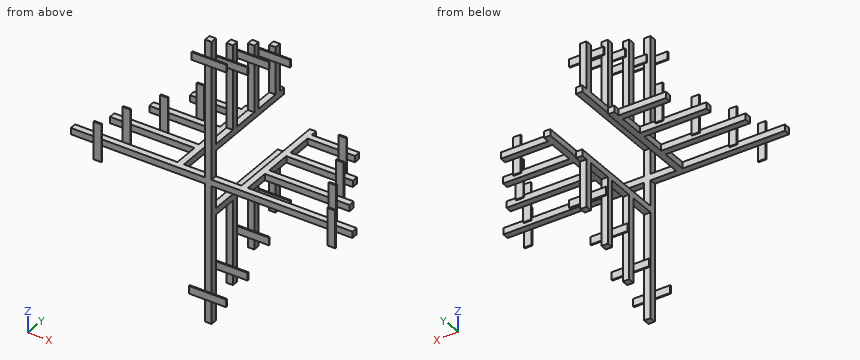
from build123d import *

# Parameters (mm, degrees)
SKETCH3_W                 = 25
SKETCH3_H                 = 25
BOSS_EXTRUDE2_DEPTH       = 550
SKETCH5_W                 = 25
SKETCH5_H                 = 25
BOSS_EXTRUDE3_DEPTH       = 550
SKETCH7_W                 = 25
SKETCH7_H                 = 25
BOSS_EXTRUDE4_DEPTH       = 400
SKETCH8_W                 = 25
SKETCH8_H                 = 25
BOSS_EXTRUDE5_DEPTH       = 400
SKETCH9_W                 = 25
SKETCH9_H                 = 25
BOSS_EXTRUDE7_DEPTH       = 260
SKETCH9_5_W               = 25
SKETCH9_5_H               = 25
BOSS_EXTRUDE8_DEPTH       = 330
SKETCH9_8_W               = 25
SKETCH9_8_H               = 25
BOSS_EXTRUDE10_DEPTH      = 185
SKETCH11_W                = 25
SKETCH11_H                = 25
BOSS_EXTRUDE11_DEPTH      = 185
SKETCH11_5_W              = 25
SKETCH11_5_H              = 25
BOSS_EXTRUDE12_DEPTH      = 260
SKETCH11_6_W              = 25
SKETCH11_6_H              = 25
BOSS_EXTRUDE13_DEPTH      = 330
SKETCH12_W                = 25
SKETCH12_H                = 25
BOSS_EXTRUDE14_DEPTH      = 185
SKETCH12_3_W              = 25
SKETCH12_3_H              = 25
BOSS_EXTRUDE15_DEPTH      = 260
SKETCH12_4_W              = 25
SKETCH12_4_H              = 25
BOSS_EXTRUDE16_DEPTH      = 330
SKETCH13_W                = 25
SKETCH13_H                = 25
BOSS_EXTRUDE17_DEPTH      = 330
SKETCH13_3_W              = 25
SKETCH13_3_H              = 25
BOSS_EXTRUDE18_DEPTH      = 260
SKETCH13_4_W              = 25
SKETCH13_4_H              = 25
BOSS_EXTRUDE19_DEPTH      = 185
BOSS_EXTRUDE21_DEPTH      = 61
BOSS_EXTRUDE21_DEPTH_BACK = 75
SKETCH15_W                = 30
SKETCH15_H                = 5
BOSS_EXTRUDE22_DEPTH      = 60
BOSS_EXTRUDE22_DEPTH_BACK = 75
SKETCH16_W                = 30
SKETCH16_H                = 5
BOSS_EXTRUDE23_DEPTH      = 61
BOSS_EXTRUDE23_DEPTH_BACK = 86
SKETCH18_W                = 30
SKETCH18_H                = 5
BOSS_EXTRUDE24_DEPTH      = 60
BOSS_EXTRUDE24_DEPTH_BACK = 85
SKETCH19_W                = 30
SKETCH19_H                = 5
BOSS_EXTRUDE27_DEPTH      = 61
BOSS_EXTRUDE27_DEPTH_BACK = 86
SKETCH20_W                = 30
SKETCH20_H                = 5


with BuildPart() as part:
    # Sketch3 → Boss-Extrude2 (new, symmetric)
    with BuildSketch(Plane.XY):
        Rectangle(SKETCH3_W, SKETCH3_H)
    extrude(amount=BOSS_EXTRUDE2_DEPTH, both=True)

    # Sketch5 → Boss-Extrude3 (add, symmetric)
    with BuildSketch(Plane(origin=(12.5, 0, 0), x_dir=(0, 0, -1), z_dir=(1, 0, 0))):
        Rectangle(SKETCH5_W, SKETCH5_H)
    extrude(amount=BOSS_EXTRUDE3_DEPTH, both=True)

    # Sketch7 → Boss-Extrude4 (add)
    with BuildSketch(Plane(origin=(0, 12.5, 0), x_dir=(1, 0, 0), z_dir=(0, 1, 0))):
        with Locations((0, -125)):
            Rectangle(SKETCH7_W, SKETCH7_H)
        with Locations((0, 125)):
            Rectangle(SKETCH7_W, SKETCH7_H)
    extrude(amount=BOSS_EXTRUDE4_DEPTH)

    # Sketch8 → Boss-Extrude5 (add)
    with BuildSketch(Plane(origin=(0, 12.5, 0), x_dir=(1, 0, 0), z_dir=(0, 1, 0))):
        with Locations((125, 0)):
            Rectangle(SKETCH8_W, SKETCH8_H)
        with Locations((-125, 0)):
            Rectangle(SKETCH8_W, SKETCH8_H)
    extrude(amount=BOSS_EXTRUDE5_DEPTH)

    # Sketch9 → Boss-Extrude7 (add)
    with BuildSketch(Plane.XY.offset(137.5)):
        with Locations((0, 250)):
            Rectangle(SKETCH9_W, SKETCH9_H)
    extrude(amount=BOSS_EXTRUDE7_DEPTH)

    # Sketch9<5> → Boss-Extrude8 (add)
    with BuildSketch(Plane.XY.offset(137.5)):
        with Locations((0, 125)):
            Rectangle(SKETCH9_5_W, SKETCH9_5_H)
    extrude(amount=BOSS_EXTRUDE8_DEPTH)

    # Sketch9<8> → Boss-Extrude10 (add)
    with BuildSketch(Plane.XY.offset(137.5)):
        with Locations((0, 375)):
            Rectangle(SKETCH9_8_W, SKETCH9_8_H)
    extrude(amount=BOSS_EXTRUDE10_DEPTH)

    # Sketch11 → Boss-Extrude11 (add)
    with BuildSketch(Plane.ZY.offset(137.5)):
        with Locations((0, 375)):
            Rectangle(SKETCH11_W, SKETCH11_H)
    extrude(amount=BOSS_EXTRUDE11_DEPTH)

    # Sketch11<5> → Boss-Extrude12 (add)
    with BuildSketch(Plane.ZY.offset(137.5)):
        with Locations((0, 250)):
            Rectangle(SKETCH11_5_W, SKETCH11_5_H)
    extrude(amount=BOSS_EXTRUDE12_DEPTH)

    # Sketch11<6> → Boss-Extrude13 (add)
    with BuildSketch(Plane.ZY.offset(137.5)):
        with Locations((0, 125)):
            Rectangle(SKETCH11_6_W, SKETCH11_6_H)
    extrude(amount=BOSS_EXTRUDE13_DEPTH)

    # Sketch12 → Boss-Extrude14 (add)
    with BuildSketch(Plane(origin=(0, 0, -137.5), x_dir=(-1, 0, 0), z_dir=(0, 0, -1))):
        with Locations((0, 375)):
            Rectangle(SKETCH12_W, SKETCH12_H)
    extrude(amount=BOSS_EXTRUDE14_DEPTH)

    # Sketch12<3> → Boss-Extrude15 (add)
    with BuildSketch(Plane(origin=(0, 0, -137.5), x_dir=(-1, 0, 0), z_dir=(0, 0, -1))):
        with Locations((0, 250)):
            Rectangle(SKETCH12_3_W, SKETCH12_3_H)
    extrude(amount=BOSS_EXTRUDE15_DEPTH)

    # Sketch12<4> → Boss-Extrude16 (add)
    with BuildSketch(Plane(origin=(0, 0, -137.5), x_dir=(-1, 0, 0), z_dir=(0, 0, -1))):
        with Locations((0, 125)):
            Rectangle(SKETCH12_4_W, SKETCH12_4_H)
    extrude(amount=BOSS_EXTRUDE16_DEPTH)

    # Sketch13 → Boss-Extrude17 (add)
    with BuildSketch(Plane(origin=(137.5, 0, 0), x_dir=(0, 0, -1), z_dir=(1, 0, 0))):
        with Locations((0, 125)):
            Rectangle(SKETCH13_W, SKETCH13_H)
    extrude(amount=BOSS_EXTRUDE17_DEPTH)

    # Sketch13<3> → Boss-Extrude18 (add)
    with BuildSketch(Plane(origin=(137.5, 0, 0), x_dir=(0, 0, -1), z_dir=(1, 0, 0))):
        with Locations((0, 250)):
            Rectangle(SKETCH13_3_W, SKETCH13_3_H)
    extrude(amount=BOSS_EXTRUDE18_DEPTH)

    # Sketch13<4> → Boss-Extrude19 (add)
    with BuildSketch(Plane(origin=(137.5, 0, 0), x_dir=(0, 0, -1), z_dir=(1, 0, 0))):
        with Locations((0, 375)):
            Rectangle(SKETCH13_4_W, SKETCH13_4_H)
    extrude(amount=BOSS_EXTRUDE19_DEPTH)

    # Sketch15 → Boss-Extrude21 (add, two sides: drawn at the far end of the back side and taken through both)
    with BuildSketch(Plane(origin=(12.5, 0, 0), x_dir=(0, 0, -1), z_dir=(1, 0, 0)).offset(-BOSS_EXTRUDE21_DEPTH_BACK)):
        with Locations((-470.519761445, -15)):
            Rectangle(SKETCH15_W, SKETCH15_H)
    extrude(amount=BOSS_EXTRUDE21_DEPTH + BOSS_EXTRUDE21_DEPTH_BACK)

    # Sketch16 → Boss-Extrude22 (add, two sides: drawn at the far end of the back side and taken through both)
    with BuildSketch(Plane(origin=(12.5, 0, 0), x_dir=(0, 0, -1), z_dir=(1, 0, 0)).offset(-BOSS_EXTRUDE22_DEPTH_BACK)):
        with Locations((-390.907976081, 110)):
            Rectangle(SKETCH16_W, SKETCH16_H)
        with Locations((-343.832488687, 235)):
            Rectangle(SKETCH16_W, SKETCH16_H)
        with Locations((-282.595194205, 360)):
            Rectangle(SKETCH16_W, SKETCH16_H)
    extrude(amount=BOSS_EXTRUDE22_DEPTH + BOSS_EXTRUDE22_DEPTH_BACK)

    # Sketch18 → Boss-Extrude23 (add, two sides: drawn at the far end of the back side and taken through both)
    with BuildSketch(Plane.XY.offset(12.5).offset(-BOSS_EXTRUDE23_DEPTH_BACK)):
        with Locations((483.727363311, -15)):
            Rectangle(SKETCH18_W, SKETCH18_H)
        with Locations((403.744811794, 110)):
            Rectangle(SKETCH18_W, SKETCH18_H)
        with Locations((349.754481778, 235)):
            Rectangle(SKETCH18_W, SKETCH18_H)
        with Locations((277.187384398, 360)):
            Rectangle(SKETCH18_W, SKETCH18_H)
    extrude(amount=BOSS_EXTRUDE23_DEPTH + BOSS_EXTRUDE23_DEPTH_BACK)

    # Sketch19 → Boss-Extrude24 (add, two sides: drawn at the far end of the back side and taken through both)
    with BuildSketch(Plane(origin=(12.5, 0, 0), x_dir=(0, 0, -1), z_dir=(1, 0, 0)).offset(-BOSS_EXTRUDE24_DEPTH_BACK)):
        with Locations((444.861975809, -15)):
            Rectangle(SKETCH19_W, SKETCH19_H)
        with Locations((409.726408873, 110)):
            Rectangle(SKETCH19_W, SKETCH19_H)
        with Locations((341.249082781, 235)):
            Rectangle(SKETCH19_W, SKETCH19_H)
        with Locations((267.100501546, 360)):
            Rectangle(SKETCH19_W, SKETCH19_H)
    extrude(amount=BOSS_EXTRUDE24_DEPTH + BOSS_EXTRUDE24_DEPTH_BACK)

    # Sketch20 → Boss-Extrude27 (add, two sides: drawn at the far end of the back side and taken through both)
    with BuildSketch(Plane(origin=(0, 0, -12.5), x_dir=(-1, 0, 0), z_dir=(0, 0, -1)).offset(-BOSS_EXTRUDE27_DEPTH_BACK)):
        with Locations((430.066631827, -15)):
            Rectangle(SKETCH20_W, SKETCH20_H)
        with Locations((400.066631827, 110)):
            Rectangle(SKETCH20_W, SKETCH20_H)
        with Locations((336.540647737, 235)):
            Rectangle(SKETCH20_W, SKETCH20_H)
        with Locations((278.06024781, 360)):
            Rectangle(SKETCH20_W, SKETCH20_H)
    extrude(amount=BOSS_EXTRUDE27_DEPTH + BOSS_EXTRUDE27_DEPTH_BACK)


solid = part.part
The model under review builds one solid part; all positions refer to its coordinate system, in mm. Give positions to 0.01 mm unless a question says otherwise; leave off trailing zeros. Write each loop counter-clockwise with the first axis right and the second up, starting at its lowest first coordinate (ties: lowest second). Pieces come first, ordered by that corner, then holes.
1. Wall thickness on L1, parallel to Y at x = -4, z = 159.5; L2, parallel to X at y = 385, z = -180; L3, parallel to Y at x = 73, z = 471.5: over which ranges is each line inside the solid? List them lowest first.
2. Add section B-B, the plane z = -165.5. Write out the cut boundary in (x, y).
3. For P1, Ø20, axis at x = -255, z = -5.5, coming from the -Y side; P2, Ø1.5, axis at y = -15.5, z = 475, coming from the -X side; P3, Ø12.5, axis at x = 4, y = 397.5, coming from the -Z side, all flat-tipped, find the tip position at first contact; note any pin that passes through.
4. Add section A-A, the plane x = -219.5. Write out the cut boundary in (y, z), plus the area to 3 significant figures.
5. Add section C-C, the plane x = -364.5. Write out the cut boundary in (y, z).
Worked answers:
1. L1: y = -12.5 to 12.5, 112.5 to 137.5, 237.5 to 262.5, 362.5 to 387.5
1. L2: x = -12.5 to 12.5
1. L3: y = -17.5 to -12.5
2. outline: (-12.5, -12.5) - (12.5, -12.5) - (12.5, 12.5) - (-12.5, 12.5) - close; (-12.5, 112.5) - (12.5, 112.5) - (12.5, 137.5) - (-12.5, 137.5) - close; (-12.5, 237.5) - (12.5, 237.5) - (12.5, 262.5) - (-12.5, 262.5) - close; (-12.5, 362.5) - (12.5, 362.5) - (12.5, 387.5) - (-12.5, 387.5) - close
3. P1: stops at y = -12.5
3. P2: stops at x = -62.5
3. P3: stops at z = -137.5
4. outline: (-12.5, -12.5) - (12.5, -12.5) - (12.5, 12.5) - (-12.5, 12.5) - close; (112.5, -12.5) - (137.5, -12.5) - (137.5, 12.5) - (112.5, 12.5) - close; (237.5, -12.5) - (262.5, -12.5) - (262.5, 12.5) - (237.5, 12.5) - close; (362.5, -12.5) - (387.5, -12.5) - (387.5, 12.5) - (362.5, 12.5) - close
4. area: 2,500 mm2
5. outline: (-12.5, -12.5) - (12.5, -12.5) - (12.5, 12.5) - (-12.5, 12.5) - close; (112.5, -12.5) - (137.5, -12.5) - (137.5, 12.5) - (112.5, 12.5) - close; (237.5, -12.5) - (262.5, -12.5) - (262.5, 12.5) - (237.5, 12.5) - close
